Read the model definition and answer for the solid it produces. Units are mm, in the model's axes. A direction names the side the tool comes from. Give positions to 0.01 mm unless a question says otherwise; leave off trailing zeros. Write each loop counter-clockwise with the first axis right and the second up, starting at its lowest first coordinate (ties: lowest second). Pieces come first, ordered by that corner, then holes. Notation, with made-up numbers: M 27,18.5 L 59,18.5 A27 ccw 59,42.5 Z; hole C 4,47.25 d3. An arc over 180 degrees is marked long. Use a Markdown table: item, result. Add a question column.
Item 1: A cutting plane is placed at A-A on z = -3.5. Determine the outline of the cut face in (x, y).
Item 2: The mould has two halves that part along Y. Classify faces 1 (the flat face through (-22, 10, -8.4)), 2 (the cylindrical face through (-17.18, 8.68, -7.33)), 3 (the cylindrical face through (-14.92, 19.892, -4.043)): pulls with the +Y half, pulls with the -Y half, needs draft (parallel to the pull), parting line crosses it, or undercut.
Item 3: Given P1, Ø2.5, axis at x = -13.5, y = 10.5, coming from the -Z side; P2, Ø0.7, axis at x = -9, z = -24, coming from the +Y side; P3, Ø4, axis at y = 6.5, z = -6.5, coming from the +X side, each flat-ended and moving along its own axis, determine where each tip first touches the part or whether it passes through.
Item 4: For faces 4 (the flat face through (-9, 10.614, -20)), 5 (the cylindrical face through (-19.228, 8.401, -20.414)), 6 (the flat face through (-18.993, 4.858, -3.057)), 7 (the flat face through (-9, 9.214, -20)), determine the directions among +Z, -Z, +X, -X, +Y, -Y from which every point of the face is accessible in a straight line to the end or side of a thin tool.
Item 5: Consider probe 1 along Z at (x, y) = (-17.75, 16); probe 2 along Y at (x, z) = (-12, -24); probe 3 along X at (y, z) = (12.75, -13). Determine where each line is inside the solid, lowest interval first. Write a range as [from, to].
Item 6: A cutting plane is placed at B-B on z = -20. Determine the outline of the cut face in (x, y).
Autodesk Inventor part; units mm, degrees
ref_plane "Work Plane1" through (0, 0, 0) normal (0, 0, 1) x (1, 0, 0)
ref_plane "YZ Plane" through (0, 0, 0) normal (1, 0, 0) x (0, 1, 0)
ref_plane "XZ Plane" through (0, 0, 0) normal (0, 1, 0) x (-1, 0, 0)
ref_plane "Work Plane1" through (0, 0, 0) normal (0, 0, 1) x (1, 0, 0)
sketch "Sketch1" plane through (0, 0, 0) normal (0, 0, 1) x (1, 0, 0)
  line L0 (-9.8058, 6.0834) -> (-16.0096, 2.999)
  line L1 (-16.0096, 2.999) -> (-21.7826, 6.8295)
  line L2 (-21.7826, 6.8295) -> (-21.3519, 13.7443)
  line L3 (-21.3519, 13.7443) -> (-15.1481, 16.8286)
  line L4 (-15.1481, 16.8286) -> (-9.3751, 12.9982)
  line L5 (-9.3751, 12.9982) -> (-9.8058, 6.0834)
  line L6 (-15.1481, 16.8286) -> (-16.0096, 2.999)
  circle A0 centre (-15.5789, 9.9138) radius 10
  point P0 (0, 0)
  dimension "d0" = 12
  dimension "d1" = 20
extrude "Extrusion1" add sketch "Sketch1" against normal blind 6.2
sketch "Sketch2" plane through (-15.5789, 9.9138, -6.2) normal (0, 0, -1) x (-1, 0, 0)
  circle A0 centre (0, 0) radius 10
  point P0 (-15.5789, -9.9138)
extrude "Extrusion2" add sketch "Sketch2" along normal blind 2.2
sketch "Sketch3" plane through (-15.5789, 9.9138, -8.4) normal (0, 0, -1) x (-1, 0, 0)
  circle A0 centre (0, 0) radius 10
  circle A1 centre (0, 0) radius 3.3
  point P0 (-15.5789, -9.9138)
  dimension "d6" = 6.6
extrude "Extrusion3" cut sketch "Sketch3" against normal through all contours A1
sketch "Sketch4" plane through (-15.5789, 9.9138, -8.4) normal (0, 0, -1) x (-1, 0, 0)
  circle A0 centre (0, 0) radius 3.3
  circle A1 centre (0, 0) radius 6.1
  point P0 (-15.5789, -9.9138)
  dimension "d9" = 12.2
extrude "Extrusion4" add sketch "Sketch4" along normal blind 23.5
chamfer "Chamfer3" distance 0.2 angle 45 1 edges at (-5.5789, 9.9138, -8.4)
sketch "Sketch6" plane through (-15.5789, 9.9138, -6.2) normal (0, 0, 1) x (1, 0, 0)
  circle A0 centre (0, 0) radius 3.3
  point P0 (15.5789, -9.9138)
extrude "Extrusion6" add sketch "Sketch6" against normal blind 2.3
sketch "Sketch7" plane through (-15.5789, 9.9138, -8.5) normal (0, 0, -1) x (-1, 0, 0)
  circle A0 centre (0, 0) radius 3.3
  circle A1 centre (0, 0) radius 1.92
  point P0 (-15.5789, -9.9138)
  dimension "d42" = 3.84
extrude "Extrusion7" cut sketch "Sketch7" against normal through all contours A1
sketch "Sketch9" plane through (-15.5789, 9.9138, -6.2) normal (0, 0, 1) x (1, 0, 0)
  circle A0 centre (0, 0) radius 1.92
  circle A1 centre (0, 0) radius 2.02
  point P0 (15.5789, -9.9138)
  dimension "d52" = 0.1
extrude "Extrusion8" cut sketch "Sketch9" against normal blind 10 contours A0 | A1
sketch "Sketch10" plane through (-15.5789, 9.9138, 0) normal (0, 0, 1) x (1, 0, 0)
  circle A0 centre (0, 0) radius 10
  line L0 (0.4308, 6.9148) -> (6.2038, 3.0844)
  line L1 (6.2038, 3.0844) -> (5.773, -3.8304)
  line L2 (5.773, -3.8304) -> (-0.4308, -6.9148)
  line L3 (-0.4308, -6.9148) -> (-6.2038, -3.0844)
  line L4 (-6.2038, -3.0844) -> (-5.773, 3.8304)
  line L5 (-5.773, 3.8304) -> (0.4308, 6.9148)
  line L6 (5.8692, -3.8943) -> (6.3072, 3.1358)
  line L7 (6.3072, 3.1358) -> (0.4379, 7.03)
  line L8 (0.4379, 7.03) -> (-5.8692, 3.8943)
  line L9 (-5.8692, 3.8943) -> (-6.3072, -3.1358)
  line L10 (-6.3072, -3.1358) -> (-0.4379, -7.03)
  line L11 (-0.4379, -7.03) -> (5.8692, -3.8943)
  point P0 (15.5789, -9.9138)
  dimension "d55" = 0.1
extrude "Extrusion9" cut sketch "Sketch10" against normal up to surface (6.2 mm away) contours L11 L10 L9 L8 L7 L6
thicken "Thicken3" operation add thickness 0.1 both sides no extend neighbours no toward (0, 0, -1) faces at (-20.6545, 9.164, -31.9) (-21.6591, 9.423, -24.0667)
sketch "Sketch11" plane through (-15.5789, 9.9138, -32) normal (0, 0, -1) x (-1, 0, 0)
  circle A0 centre (0, 0) radius 6.2
  circle A1 centre (0, 0) radius 6.2
  line L0 (-6.2, 0) -> (-6.2, 0.7)
  line L1 (-6.2, 0) -> (-5.5, 0) construction
  line L2 (-6.2, 0) -> (-6.2, -0.7)
  line L3 (-6.2, 0) -> (-5.5, 0) construction
  line L4 (-6.2, 0) -> (-6.7, 0)
  line L5 (-6.75, -0.7) -> (-5.75, -0.7)
  line L6 (-5.75, -0.7) -> (-5.75, 0.7)
  line L7 (-5.75, 0.7) -> (-6.75, 0.7)
  line L8 (-6.75, 0.7) -> (-6.75, -0.7)
  point P0 (-15.5789, -9.9138)
  dimension "d60" = 0.7
  dimension "d61" = 90
  dimension "d62" = 0.7
  dimension "d63" = 90
  dimension "d64" = 0.5
  dimension "d79" = 1
  dimension "d80" = 5.75
extrude "Extrusion10" add sketch "Sketch11" against normal up to surface (23.6 mm away) contours L7 L6 L5 A0 | A0 L0 L7 | L5 L2 A0 | L2 L5 L8 L7 L0 picked at (-5.9, 0)
chamfer "Chamfer9" distance 0.3 angle 45 2 edges at (-15.9294, 3.7237, -32) (-15.9294, 16.1039, -32)
chamfer "Chamfer10" distance 0.3 angle 45 1 edges at (-8.8289, 9.9138, -32)
sketch "Sketch14" plane through (-15.5789, 9.9138, -32) normal (0, 0, -1) x (-1, 0, 0)
  line L0 (-6.45, -0.7) -> (-6.45, 0.7)
  line L1 (-6.45, -0.7) -> (-5.8583, -0.7)
  arc A0 (-5.8583, -0.7) -> (-5.8583, 0.7) centre (0, 0) ccw
  line L2 (-5.8583, 0.7) -> (-6.45, 0.7)
  circle A1 centre (0, 0) radius 3.3
  circle A2 centre (0, 0) radius 3.95
  point P0 (-15.5789, -9.9138)
  dimension "d75" = 6.6
  dimension "d76" = 7.9
extrude "Extrusion12" cut sketch "Sketch14" against normal up to surface (23.5 mm away) contours A1 | A2
properties part number "omni_ext_3DPrint"
Filled in:
| question | item | result |
|---|---|---|
| 1 | outline | C -15.58,9.91 d20; hole M -21.89,6.78 L -16.02,2.88 L -9.71,6.02 L -9.27,13.05 L -15.14,16.94 L -21.45,13.81 Z |
| 2 | face 1 | needs draft |
| 2 | face 2 | undercut |
| 2 | face 3 | parting line crosses it |
| 3 | P1 | z = -8.5 |
| 3 | P2 | y = 10.61 |
| 3 | P3 | x = -5.68 |
| 4 | face 4 | -Z, +X, +Y |
| 4 | face 5 | -Z |
| 4 | face 6 | +Z |
| 4 | face 7 | -Z, +X, -Y |
| 5 | probe 1 | [-8.4, 0] |
| 5 | probe 2 | [4.85, 8.24], [11.59, 14.98] |
| 5 | probe 3 | [-21.09, -18.33], [-12.83, -10.07] |
| 6 | outline | M -9.42,9.21 L -8.83,9.21 L -8.83,10.61 L -9.42,10.61 A6.2 ccw long Z; hole C -15.58,9.91 d7.9 |
